from build123d import *

# Parameters (mm, degrees)
F0_W     = 138.403788
F0_H     = 93.97047
F1_DEPTH = 38.1
F3_DEPTH = 57.15
F4_R     = 27.26818
F5_DEPTH = 63.5
F6_R     = 9.867741
F7_DEPTH = 203.2


with BuildPart() as f1:
    # F0 (on Right) → F1 (new body, symmetric)
    with BuildSketch(Plane.YZ):
        Rectangle(F0_W, F0_H)
    extrude(amount=F1_DEPTH, both=True)

    # F2 (on Right) → F3 (join, symmetric)
    with BuildSketch(Plane.YZ):
        with BuildLine():
            Line((39.828518, 46.985235), (-39.828518, 46.985235))
            ThreePointArc((-39.828518, 46.985235), (0, 7.156717), (39.828518, 46.985235))
        make_face()
    extrude(amount=F3_DEPTH, both=True)

    # F4 (on Right) → F5 (cut, symmetric)
    with BuildSketch(Plane.YZ):
        with Locations((0, 46.985235)):
            Circle(F4_R)
    extrude(amount=F5_DEPTH, both=True, mode=Mode.SUBTRACT)

    # F6 (on face) → F7 (cut)
    with BuildSketch(Plane.XY.offset(46.985235)):
        with Locations((0, 49.696259)):
            Circle(F6_R)
        with Locations((0, -49.696259)):
            Circle(F6_R)
    extrude(amount=-F7_DEPTH, mode=Mode.SUBTRACT)


solid = f1.part
Geometry check sheet. Reference: the model listing, model coordinates, mm. A direction names the side the tool comes from. Round coordinates to 2 decimals unless told otherwise and drop trailing zeros. Loops run counter-clockwise (first coordinate to the right, second up) from the corner with the lowest first, then second, coordinate; pieces in that order, holes last. Notation, with made-up numbers: (30.25, 23) - (86.25, 23) arc R19 ccw to (86.25, 48) - close; hole circle Ø7 at (6.25, 51). An arc over 180 degrees is marked (long way). One line per question, with ' | ' between items. Start each with the question number.
1. Cross-section at D-D on z = 13. Record the cut outline in (x, y).
2. Draft check along X on faces 1 (the face through (47.758, -0.876, 7.166)), 2 (the face through (57.15, -1, 18)), 3 (the face through (5.3, 58.02, 0.66)). Enter one of: released by +X, released by -X, zero draft, split by the parting line, or undercut.
3. Scan lines: line 1 (Y direction, x = 0, z = 10); line 2 (Y direction, x = 0, z = 26.5); line 3 (X direction, y = 18, z = 0.5). Record each from-to range of solid material in increasing order. Write a range as [from, to].
4. Tool access check on faces 4 (the face through (1, -1, -46.985)), 5 (the face through (-38.1, -1, -10)), 6 (the face through (38.1, -1, -10)). Record the directions out of +Z, -Z, +X, -X, +Y, -Y that give a thin tool (end or side, any length) a straight path to the whole face; none if there is none.
5. Depth check by flat-ended pin: pin 1 (10 mm diameter, centred on y = 45, z = -10, fed in from +X). Enter the tip coordinate at first touch or a pass-through.
6. Cross-section at A-A on x = 0. Record the cut outline in (y, z).
7. Cross-section at C-C on y = 0. Record the cut outline in (x, z), then the cut area to 3 significant figures.
8. Cross-section at B-B on z = 31.5. Record the cut outline in (x, y), then the cut area to 3 significant figures.
Taken from the geometry:
1) outline: (-57.15, -20.77) - (-38.1, -20.77) - (-38.1, -69.2) - (38.1, -69.2) - (38.1, -20.77) - (57.15, -20.77) - (57.15, 20.77) - (38.1, 20.77) - (38.1, 69.2) - (-38.1, 69.2) - (-38.1, 20.77) - (-57.15, 20.77) - close; hole circle Ø19.74 at (0, -49.7); hole circle Ø19.74 at (0, 49.7)
2) face 1: zero draft | face 2: released by +X | face 3: undercut
3) line 1: [-69.2, -59.56], [-39.83, 39.83], [59.56, 69.2] | line 2: [-69.2, -59.56], [-39.83, -18], [18, 39.83], [59.56, 69.2] | line 3: [-38.1, 38.1]
4) face 4: -Z, +X, -X, +Y, -Y | face 5: -Z, -X | face 6: -Z, +X
5) pin 1: x = 38.1
6) outline: (-69.2, -46.99) - (-59.56, -46.99) - (-59.56, 46.99) - (-69.2, 46.99) - close; (-39.83, -46.99) - (39.83, -46.99) - (39.83, 46.99) - (27.27, 46.99) arc R27.27 cw to (-27.27, 46.99) - (-39.83, 46.99) - close; (59.56, -46.99) - (69.2, -46.99) - (69.2, 46.99) - (59.56, 46.99) - close
7) outline: (-57.15, 7.16) - (-38.1, 7.16) - (-38.1, -46.99) - (38.1, -46.99) - (38.1, 7.16) - (57.15, 7.16) - (57.15, 19.72) - (-57.15, 19.72) - close | area: 5,560 mm²
8) outline: (-57.15, -36.69) - (-38.1, -36.69) - (-38.1, -69.2) - (38.1, -69.2) - (38.1, -36.69) - (57.15, -36.69) - (57.15, -22.44) - (-57.15, -22.44) - close; (-57.15, 22.44) - (57.15, 22.44) - (57.15, 36.69) - (38.1, 36.69) - (38.1, 69.2) - (-38.1, 69.2) - (-38.1, 36.69) - (-57.15, 36.69) - close; hole circle Ø19.74 at (0, -49.7); hole circle Ø19.74 at (0, 49.7) | area: 7,600 mm²
